Work out the finished part from the listing and answer in its coordinate system (mm). A direction names the side the tool comes from. Give positions to 0.01 mm unless a question says otherwise; leave off trailing zeros. Write each loop counter-clockwise with the first axis right and the second up, starting at its lowest first coordinate (ties: lowest second). Pieces come first, ordered by that corner, then holes. Notation, with made-up numbers: (40, 9) -> (76, 9) arc R32 cw to (76, 46) -> close; hole circle Ø11 at (54.5, -24). An arc over 180 degrees is marked (long way). Use a Markdown table: item, result. Add a question column.
Q1. Consider line 1 (Z direction, x = 79, y = 21) (3 decimals); line 2 (X direction, y = 20.5, z = 0.5); line 3 (X direction, y = 23, z = -6.5). Determine where each line is inside the solid, lowest interval first.
Q2. For faces 1 (the face through (-20.49, -3.33, 1.57)), 2 (the face through (11.12, 23.59, -2.89)), 3 (the face through (-5.571, 10.992, -6.261)), 4 (the face through (-3, 14, -12.7)), determine the directions among +Z, -Z, +X, -X, +Y, -Y from which every point of the face is accessible in a straight line to the end or side of a thin tool.
Q3. For a pull along X with two mould halves and no side action, classify faces 5 (the face through (152.911, 11, 2)), 6 (the face through (19.4, 24.6, 1.6)), 7 (the face through (-3.98, 14.02, -3.32)), 8 (the face through (88, 28.9, 2)) as pulls with the +X half, pulls with the -X half, needs draft (parallel to the pull), parting line crosses it, or undercut.
Q4. Section B-B, the plane x = 128.5 is taken. Give the vertices of the cut face in (y, z) (3 decimals), plus the area to 3 significant figures.
Q5. Section A-A, the plane z = -5 is taken. Give the vertices of the cut face in (x, y), plus the area to 3 significant figures.
Q6. Each of these flat-tipped pins is pushed along its axis until it touches: pin 1 Ø6 at (y, z) = (3.5, -8.5) entering from -X; pin 2 Ø4 at (x, y) = (86.5, 10.5) entering from -Z. Where does it stop, or does it pass through?
Q7. Section C-C, the plane y = -0.5 is taken. Give the vertices of the cut face in (x, z) (3 decimals).
Autodesk Inventor part; units mm, degrees
ref_plane "YZ Plane" through (0, 0, 0) normal (1, 0, 0) x (0, 1, 0)
ref_plane "XZ Plane" through (0, 0, 0) normal (0, 1, 0) x (-1, 0, 0)
ref_plane "XY Plane" through (0, 0, 0) normal (0, 0, 1) x (1, 0, 0)
sketch "Sketch1" plane through (0, 0, 0) normal (0, 0, 1) x (1, 0, 0)
  line L0 (-26.4763, -7.5222) -> (152.9112, -7.5222)
  line L1 (-26.4763, -7.5222) -> (25.5399, 28.8999)
  line L2 (-26.4763, -7.5222) -> (37.0237, -7.5222) construction
  line L3 (25.5399, 28.8999) -> (152.9112, 28.8999)
  line L4 (152.9112, 28.8999) -> (152.9112, -7.5222)
  point P0 (0, 0)
  dimension "d0" = 179.3875
  dimension "d2" = 63.5
  dimension "d3" = 35
extrude "Extrusion1" add sketch "Sketch1" along normal blind 3.175
sketch "Sketch2" plane through (0, 0, 0) normal (0, 0, -1) x (-1, 0, 0)
  line L0 (-25.5399, 28.8999) -> (26.4763, -7.5222)
  line L1 (0.4682, 10.6889) -> (-13.3681, 20.3771)
  line L2 (-13.3681, 20.3771) -> (-9.7259, 25.5788)
  line L3 (-9.7259, 25.5788) -> (17.9675, 6.1876)
  line L4 (17.9675, 6.1876) -> (14.3253, 0.986)
  line L5 (14.3253, 0.986) -> (0.4682, 10.6889)
  point P0 (0, 0)
  dimension "d6" = 16.891
  dimension "d7" = 6.35
  dimension "d8" = 33.8074
extrude "Extrusion2" add sketch "Sketch2" against normal blind 3.175
sketch "Sketch3" plane through (0, 0, 0) normal (0, 0, -1) x (-1, 0, 0)
  line L0 (14.3253, 0.986) -> (17.9675, 6.1876)
  line L1 (17.9675, 6.1876) -> (-9.7259, 25.5788)
  line L2 (-9.7259, 25.5788) -> (-13.3681, 20.3771)
  line L3 (-25.5399, 28.8999) -> (-13.3681, 20.3771)
  line L4 (-9.7259, 25.5788) -> (17.9675, 6.1876)
  line L5 (17.9675, 6.1876) -> (16.1464, 3.5868)
  line L6 (16.1464, 3.5868) -> (-11.547, 22.9779)
  line L7 (-11.547, 22.9779) -> (-9.7259, 25.5788)
  point P0 (0, 0)
  dimension "d11" = 3.175
extrude "Extrusion3" add sketch "Sketch3" along normal blind 12.7
sketch "Sketch4" plane through (-17.9675, 6.1876, 3.175) normal (-0.5736, 0.8192, 0) x (0.8192, 0.5736, 0)
  line L0 (0, 15.875) -> (33.8074, 15.875)
  line L1 (16.9037, 15.875) -> (16.9037, 9.525)
  point P0 (11.1691, 3.175)
  dimension "d14" = 6.35
hole "Hole1" at (-4.1208, 15.8832, -6.35) direction (0.5736, -0.8192, 0) diameter 6.35 end through all
properties part number "Right Forearm"
Result set:
| question | item | result |
|---|---|---|
| 1 | line 1 | z = 0 to 3.175 |
| 1 | line 2 | x = 2.47 to 13.28, 13.54 to 152.91 |
| 1 | line 3 | x = 6.04 to 11.53 |
| 2 | face 1 | +Z, -Z, -X |
| 2 | face 2 | +Z, -Z, +Y |
| 2 | face 3 | -Z, +X, -Y |
| 2 | face 4 | -Z, +X, -X, +Y, -Y |
| 3 | face 5 | pulls with the +X half |
| 3 | face 6 | undercut |
| 3 | face 7 | undercut |
| 3 | face 8 | needs draft |
| 4 | outline | (-7.522, 0) -> (28.9, 0) -> (28.9, 3.175) -> (-7.522, 3.175) -> close |
| 4 | area | 116 mm2 |
| 5 | outline | (-17.97, 6.19) -> (-16.15, 3.59) -> (-4.65, 11.63) -> (-6.47, 14.23) -> close; (-1.77, 17.53) -> (0.05, 14.93) -> (11.55, 22.98) -> (9.73, 25.58) -> close |
| 5 | area | 89.1 mm2 |
| 6 | pin 1 | stops at x = -17.97 |
| 6 | pin 2 | stops at z = 0 |
| 7 | outline | (-16.448, 0) -> (152.911, 0) -> (152.911, 3.175) -> (-16.448, 3.175) -> close |
